```python
from build123d import *

# Parameters (mm, degrees)
F0_R     = 24.5
F0_R_2   = 12.5
F1_DEPTH = 15
F2_DEPTH = 25
F3_R     = 3
F4_SIZE  = 3


# Not quite as in the source:
# - a feature names something its author has since deleted; it is built from what else it names


with BuildPart() as f1:
    # F0 (on Top) → F1 (new body)
    with BuildSketch(Plane.XY):
        with BuildLine():
            ThreePointArc((35, 0), (26.4758800085, 22.8916530154), (5.0555555556, 34.6329519104))
            ThreePointArc((5.0555555556, 34.6329519104), (-35, 0), (5.0555555556, -34.6329519104))
            ThreePointArc((5.0555555556, -34.6329519104), (26.4758800085, -22.8916530154), (35, 0))
        make_face()
        Circle(F0_R, mode=Mode.SUBTRACT)
        with BuildLine():
            Line((93.1777777778, 21.7692840579), (5.0555555556, 34.6329519104))
            ThreePointArc((5.0555555556, 34.6329519104), (26.4758800085, 22.8916530154), (35, 0))
            ThreePointArc((35, 0), (26.4758800085, -22.8916530154), (5.0555555556, -34.6329519104))
            Line((5.0555555556, -34.6329519104), (93.1777777778, -21.7692840579))
            ThreePointArc((93.1777777778, -21.7692840579), (68, 0), (93.1777777778, 21.7692840579))
        make_face()
        with BuildLine():
            ThreePointArc((112, 0), (106.6419817196, 14.3890390383), (93.1777777778, 21.7692840579))
            ThreePointArc((93.1777777778, 21.7692840579), (68, 0), (93.1777777778, -21.7692840579))
            ThreePointArc((93.1777777778, -21.7692840579), (106.6419817196, -14.3890390383), (112, 0))
        make_face()
        with Locations((90, 0)):
            Circle(F0_R_2, mode=Mode.SUBTRACT)
    extrude(amount=-F1_DEPTH)

    # F0 (on Top) → F2 (join)
    with BuildSketch(Plane.XY):
        with BuildLine():
            ThreePointArc((35, 0), (26.4758800085, 22.8916530154), (5.0555555556, 34.6329519104))
            ThreePointArc((5.0555555556, 34.6329519104), (-35, 0), (5.0555555556, -34.6329519104))
            ThreePointArc((5.0555555556, -34.6329519104), (26.4758800085, -22.8916530154), (35, 0))
        make_face()
        Circle(F0_R, mode=Mode.SUBTRACT)
    extrude(amount=F2_DEPTH)

    # F3
    f3_edges = [f1.edges().sort_by_distance(p)[0] for p in [
        (-5.055556, 34.632952, 25),
        (-24.5, 0, 25),
        (-35, 0, -15),
        (49.116667, -28.201118, -15),
        (112, 0, -15),
        (49.116667, 28.201118, -15),
        (-24.5, 0, -15),
        (77.5, 0, -15),
    ]]
    fillet(f3_edges, radius=F3_R)

    # F4
    f4_edges = [f1.edges().sort_by_distance(p)[0] for p in [
        (77.5, 0, 0),
    ]]
    chamfer(f4_edges, length=F4_SIZE)


solid = f1.part
```
The model under review builds one solid part; all positions refer to its coordinate system, in mm. Round coordinates to 2 decimals unless told otherwise and drop trailing zeros. Loops run counter-clockwise (first coordinate to the right, second up) from the corner with the lowest first, then second, coordinate; pieces in that order, holes last.
Item 1: For line 1 (X direction, y = 4.5, z = -3.5); line 2 (Z direction, x = 62, y = 16); line 3 (X direction, y = -11, z = 16.5), list the stretches that pass through material, from the lowest coordinate up.
Determined:
line 1: x = -34.71 to -24.08, 24.08 to 78.34, 101.66 to 111.53
line 2: z = -15 to 0
line 3: x = -33.23 to -21.89, 21.89 to 33.23
Item 2: Mouldability with a two-part tool opening along Y and no side actions: class faces 1 (the face through (101.923, 3.755, -7.437)), 2 (the face through (48.5, -28.29, -5.92)), 3 (the face through (49.73, 28.11, -5.92)) as released by +Y, released by -Y, zero draft, split by the parting line, or undercut.
Determined:
face 1: undercut
face 2: released by -Y
face 3: released by +Y
Item 3: Take a section at C-C (y = 2). Give the number of separate pieces and of enclosed holes in the cut face, then the cut area to 3 significant figures.
Determined:
separate pieces: 3
enclosed holes: 0
area: 1,600 mm2
Item 4: Take a section at B-B (z = 19). Write out the cut boundary in (x, y).
Determined:
outline: circle Ø70 at (0, 0); hole circle Ø49 at (0, 0)
Item 5: Take a section at A-A (z = -9). Write out the cut boundary in (x, y), then the cut area to 3 significant figures.
Determined:
outline: (5.06, -34.63) - (93.18, -21.77) arc R22 ccw to (93.18, 21.77) - (5.06, 34.63) arc R35 ccw (long way) to start; hole circle Ø49 at (0, 0); hole circle Ø25 at (90, 0)
area: 5,490 mm2
Item 6: Clearance check with flat-ended pins moving along their axes: pin 1 Ø12 at (y, z) = (-15.5, 12.5) entering from +X; pin 2 Ø1 at (y, z) = (9, -11) entering from +X; pin 3 Ø10 at (y, z) = (-19.5, 2.5) entering from +X. State where each tip first meets the part, or that it passes through.
Determined:
pin 1: stops at x = 33.69
pin 2: stops at x = 110.29
pin 3: stops at x = 105.93
